from build123d import *

# Parameters (mm, degrees)
SKETCH1_W                = 39.5
SKETCH1_H                = 16.2
BOSS_EXTRUDE1_DEPTH      = 1.6
F_3_0_3_DIAMETER_HOLE1_D = 3
SKETCH4_W                = 12.85
SKETCH4_H                = 7
BOSS_EXTRUDE2_DEPTH      = 6
SKETCH5_W                = 14
SKETCH5_H                = 12.5
BOSS_EXTRUDE3_DEPTH      = 5.25
SKETCH6_W                = 3.75
SKETCH6_H                = 7.8
BOSS_EXTRUDE4_DEPTH      = 1.5
SKETCH7_W                = 1.65
SKETCH7_H                = 3
BOSS_EXTRUDE5_DEPTH      = 3
BOSS_EXTRUDE6_START      = -1.25
BOSS_EXTRUDE6_DEPTH      = 3.6
SKETCH13_W               = 2
SKETCH13_H               = 2.25
CUT_EXTRUDE5_DEPTH       = 26.933403936
SKETCH10_W               = 1.5
SKETCH10_H               = 5.4
CUT_EXTRUDE2_DEPTH       = 2.5
SKETCH11_W               = 0.75
SKETCH11_H               = 5.2
CUT_EXTRUDE3_DEPTH       = 43.39742256
CUT_EXTRUDE4_DEPTH       = 12


with BuildPart() as part:
    # Sketch1 → Boss-Extrude1 (new body)
    with BuildSketch(Plane.XY):
        Rectangle(SKETCH1_W, SKETCH1_H)
    extrude(amount=-BOSS_EXTRUDE1_DEPTH)

    # Ø3.0 (3) Diameter Hole1 (through all)
    with Locations(Plane.XY):
        with Locations((-2.5, 5.1), (16.25, 5.1)):
            Hole(F_3_0_3_DIAMETER_HOLE1_D / 2)

    # Sketch4 → Boss-Extrude2 (add)
    with BuildSketch(Plane.XY):
        with Locations((6.575, 4.6)):
            Rectangle(SKETCH4_W, SKETCH4_H)
    extrude(amount=BOSS_EXTRUDE2_DEPTH)

    # Sketch5 → Boss-Extrude3 (add)
    with BuildSketch(Plane.XY):
        with Locations((-14.75, 0)):
            Rectangle(SKETCH5_W, SKETCH5_H)
    extrude(amount=BOSS_EXTRUDE3_DEPTH)

    # Sketch6 → Boss-Extrude4 (add)
    with BuildSketch(Plane.XY.offset(5.25)):
        with Locations((-19.875, 0)):
            Rectangle(SKETCH6_W, SKETCH6_H)
    extrude(amount=BOSS_EXTRUDE4_DEPTH)

    # Sketch7 → Boss-Extrude5 (add)
    with BuildSketch(Plane.XY):
        with Locations((11.825, -0.4)):
            Rectangle(SKETCH7_W, SKETCH7_H)
        with Locations((6.575, -0.4)):
            Rectangle(SKETCH7_W, SKETCH7_H)
        with Locations((1.325, -0.4)):
            Rectangle(SKETCH7_W, SKETCH7_H)
    extrude(amount=BOSS_EXTRUDE5_DEPTH)

    # Sketch8 → Boss-Extrude6 (add)
    with BuildSketch(Plane(origin=(0, 0, 0), x_dir=(-1, 0, 0), z_dir=(0, 0, -1)).offset(BOSS_EXTRUDE6_START)):
        Polygon((-13, 11.261122396), (-0.555210526, 8.1), (-0.15, 8.1), (-13, 11.485488222), align=None)
    extrude(amount=-BOSS_EXTRUDE6_DEPTH)

    # Sketch13 → Cut-Extrude5 (cut, through all)
    with BuildSketch(Plane.ZY.offset(-0.5)):
        with Locations((1, -0.025)):
            Rectangle(SKETCH13_W, SKETCH13_H)
    extrude(amount=-CUT_EXTRUDE5_DEPTH, mode=Mode.SUBTRACT)

    # Sketch10 → Cut-Extrude2 (cut)
    with BuildSketch(Plane(origin=(-18, 0, 0), x_dir=(0, 0, -1), z_dir=(1, 0, 0))):
        with Locations((-6, 0)):
            Rectangle(SKETCH10_W, SKETCH10_H)
    extrude(amount=-CUT_EXTRUDE2_DEPTH, mode=Mode.SUBTRACT)

    # Sketch11 → Cut-Extrude3 (cut, through all)
    with BuildSketch(Plane(origin=(-20.5, 0, 0), x_dir=(0, 0, -1), z_dir=(1, 0, 0))):
        with Locations((-5.625, 0)):
            Rectangle(SKETCH11_W, SKETCH11_H)
    extrude(amount=-CUT_EXTRUDE3_DEPTH, mode=Mode.SUBTRACT)

    # Sketch12 → Cut-Extrude4 (cut)
    with BuildSketch(Plane(origin=(-21.75, 0, 0), x_dir=(0, 0, -1), z_dir=(1, 0, 0))):
        Polygon((-6, -2.6), (-4.7, -2.6), (-4.7, -4.95), (-2.05, -4.95), (-2.05, 4.95), (-4.7, 4.95), (-4.7, 2.6), (-6, 2.6), align=None)
    extrude(amount=CUT_EXTRUDE4_DEPTH, mode=Mode.SUBTRACT)


solid = part.part
Work out the finished part from the listing and answer in its coordinate system (mm). A direction names the side the tool comes from. Round coordinates to 2 decimals unless told otherwise and drop trailing zeros. Write each loop counter-clockwise with the first axis right and the second up, starting at its lowest first coordinate (ties: lowest second). Pieces come first, ordered by that corner, then holes.
1) A cutting plane is placed at B-B (y = 0.25). Give the vertices of the cut face in (x, z).
2) A cutting plane is placed at D-D (x = 8). Give the vertices of the cut face in (y, z), plus the area to 3 significant figures.
3) A cutting plane is placed at A-A (x = -2.5). Give the vertices of the cut face in (y, z).
4) Straight lines are drawn through the part: line 1 (Y direction, x = -2.5, z = -0.7); line 2 (Y direction, x = -11, z = 4.75); line 3 (Z direction, x = 7, y = -7). For each, find the intervals that lie inside material, in ascending order.
5) A tool of negligible diameter and unlimited length cuts with its end or side. For faces 1 (the flat face through (-20, 3.9, 6)), 2 (the flat face through (7, -1.9, 1)), 3 (the flat face through (6, 1.1, 4)), 4 (the flat face through (-19, 2.7, 6)), from which of +Z, -Z, +X, -X, +Y, -Y can it reach the whole face along a straight path? Write none if from no direction.
6) Given pin 1 Ø1 at (y, z) = (3, 1) entering from +X; pin 2 Ø1.6 at (y, z) = (-2, 2.5) entering from +X; pin 3 Ø3 at (x, z) = (-16, -0.5) entering from +Y, each flat-ended and moving along its own axis, determine where each tip first touches the part or whether it passes through.
7) A cutting plane is placed at C-C (y = 5.75). Give the vertices of the cut face in (x, z), plus the area to 3 significant figures.
8) The mould has two halves that part along Y. Classify faces 5 (the flat face through (-15, -6.25, 3)), 6 (the flat face through (-16, 0, 2.05)), 7 (the flat face through (1, 0, 2)), 8 (the flat face through (-21, 0, 0)): pulls with the +Y half, pulls with the -Y half, needs draft (parallel to the pull), parting line crosses it, or undercut.
Completed:
1. outline: (-21.75, 0) - (-19.75, 0) - (-19.75, -1.6) - (19.75, -1.6) - (19.75, 0) - (-7.75, 0) - (-7.75, 5.25) - (-9.75, 5.25) - (-9.75, 2.05) - (-21.75, 2.05) - close; (-21.75, 6) - (-20.5, 6) - (-20.5, 6.75) - (-21.75, 6.75) - close; (0.5, 2) - (2.15, 2) - (2.15, 3) - (0.5, 3) - close; (5.75, 2) - (7.4, 2) - (7.4, 3) - (5.75, 3) - close; (11, 2) - (12.65, 2) - (12.65, 3) - (11, 3) - close
2. outline: (-8.1, -1.6) - (8.1, -1.6) - (8.1, 6) - (1.1, 6) - (1.1, 0) - (-8.1, 0) - close; (9.99, 1.25) - (10.17, 1.25) - (10.17, 4.85) - (9.99, 4.85) - close
2. area: 68.6 mm2
3. outline: (-8.1, -1.6) - (3.6, -1.6) - (3.6, 0) - (-8.1, 0) - close; (6.6, -1.6) - (8.1, -1.6) - (8.1, 0) - (6.6, 0) - close
4. line 1: y = -8.1 to 3.6, 6.6 to 8.1
4. line 2: y = -6.25 to -2.6, 2.6 to 6.25
4. line 3: z = -1.6 to 0
5. face 1: +Z, -X, +Y
5. face 2: +Z, +X, -Y
5. face 3: none
5. face 4: +Z
6. pin 1: stops at x = 13
6. pin 2: stops at x = 12.65
6. pin 3: stops at y = 8.1
7. outline: (-21.75, 0) - (-19.75, 0) - (-19.75, -1.6) - (-3.85, -1.6) - (-3.85, 0) - (-7.75, 0) - (-7.75, 5.25) - (-21.75, 5.25) - close; (-1.15, -1.6) - (14.9, -1.6) - (14.9, 0) - (13, 0) - (13, 6) - (0.15, 6) - (0.15, 0) - (-1.15, 0) - close; (17.6, -1.6) - (19.75, -1.6) - (19.75, 0) - (17.6, 0) - close
7. area: 205 mm2
8. face 5: pulls with the -Y half
8. face 6: undercut
8. face 7: undercut
8. face 8: needs draft
